from build123d import *

# Parameters (mm, degrees)
SKETCH_1_W      = 70
SKETCH_1_H      = 50
SKETCH_1_R      = 15.5
EXTRUDE_1_DEPTH = 18
SKETCH_2_R      = 15.5
EXTRUDE_2_DEPTH = 2


with BuildPart() as part:
    # 草图1 → 凸台-拉伸1 (new body)
    with BuildSketch(Plane.XY):
        with Locations((35, 25)):
            Rectangle(SKETCH_1_W, SKETCH_1_H)
        with Locations((35, 25)):
            Circle(SKETCH_1_R, mode=Mode.SUBTRACT)
    extrude(amount=EXTRUDE_1_DEPTH)

    # 草图2 → 凸台-拉伸2 (add)
    with BuildSketch(Plane.XY):
        with Locations((35, 25)):
            Circle(SKETCH_2_R)
    extrude(amount=EXTRUDE_2_DEPTH)


solid = part.part
Design review of the part built by this model. Coordinates are the model's own, in mm. A direction names the side the tool comes from. Round coordinates to 2 decimals unless told otherwise and drop trailing zeros. Loops run counter-clockwise (first coordinate to the right, second up) from the corner with the lowest first, then second, coordinate; pieces in that order, holes last. Notation, with made-up numbers: (60.5, -24.5) - (85.5, -24.5) arc R11 ccw to (85.5, -5.5) - close; hole circle Ø3 at (89, 45.25). An arc over 180 degrees is marked (long way). One line per item, written item: value. Start each with the question number.
1) Consider section A-A on y = 25. Give the boundary of the cut face in (x, z).
2) Consider section C-C on x = 35. Give the boundary of the cut face in (y, z).
3) For faces 5 (the flat face through (70, 25, 9)), 6 (the cylindrical face through (43.33, 38.07, 9.89)), list the 3-axis set-ups (+Z, -Z, +X, -X, +Y, -Y) from which the entire face can be reached by the end or side of a thin tool; tool diameter is ignored.
4) Draft analysis for pull direction Y (two halves, no side actions). For faces 1 (the flat face through (35, 50, 9)), 2 (the flat face through (35, 25, 2)), 3 (the flat face through (35, 0, 9)), 4 (the flat face through (35, 25, 0)), state which applies: +Y half, -Y half, draft (parallel to the pull), parting line (faces both ways), or undercut.
5) To check wall thickness, follow L1, parallel to Y at x = 35, z = 10.5; L2, parallel to Z at x = 37, y = 38.5; L3, parallel to X at y = 11, z = 12.25. State the ranges of each line that lie inside material, in increasing order. Write a range as from..to.
6) Consider section B-B on z = 3. Give the boundary of the cut face in (x, y), then the cut area to 3 significant figures.
Reported:
1. outline: (0, 0) - (70, 0) - (70, 18) - (50.5, 18) - (50.5, 2) - (19.5, 2) - (19.5, 18) - (0, 18) - close
2. outline: (0, 0) - (50, 0) - (50, 18) - (40.5, 18) - (40.5, 2) - (9.5, 2) - (9.5, 18) - (0, 18) - close
3. face 5: +Z, -Z, +X, +Y, -Y
3. face 6: +Z
4. face 1: +Y half
4. face 2: undercut
4. face 3: -Y half
4. face 4: draft
5. L1: y = 0..9.5, 40.5..50
5. L2: z = 0..2
5. L3: x = 0..28.35, 41.65..70
6. outline: (0, 0) - (70, 0) - (70, 50) - (0, 50) - close; hole circle Ø31 at (35, 25)
6. area: 2,750 mm^2
